Autodesk Inventor part; units mm, degrees
ref_plane "YZ Plane" through (0, 0, 0) normal (1, 0, 0) x (0, 1, 0)
ref_plane "XZ Plane" through (0, 0, 0) normal (0, 1, 0) x (-1, 0, 0)
ref_plane "XY Plane" through (0, 0, 0) normal (0, 0, 1) x (1, 0, 0)
sketch "Эскиз1" plane through (0, 0, 0) normal (0, 1, 0) x (-1, 0, 0)
  line L0 (2.54, -1.27) -> (-2.54, -1.27)
  line L1 (-2.54, -1.27) -> (-2.54, 1.27)
  line L2 (-2.54, 1.27) -> (2.54, 1.27)
  line L3 (2.54, 1.27) -> (2.54, -1.27)
  line L4 (0, -1.778) -> (0, 1.778)
  line L5 (3.556, 0) -> (-3.556, 0)
  point P0 (0, 0)
  dimension "d0" = 5.08
  dimension "d1" = 2.54
extrude "Выдавливание1" add sketch "Эскиз1" along normal blind 6
sketch "Эскиз2" plane through (0, 6, 0) normal (0, 1, 0) x (1, 0, 0)
  line L0 (-1.67, 0.4) -> (-0.87, 0.4)
  line L1 (-0.87, 0.4) -> (-0.87, -0.4)
  line L2 (-0.87, -0.4) -> (-1.67, -0.4)
  line L3 (-1.67, -0.4) -> (-1.67, 0.4)
  line L4 (-3.556, 0) -> (3.556, 0)
  line L5 (0, 1.778) -> (0, -1.778)
  line L6 (0.87, 0.4) -> (1.67, 0.4)
  line L7 (1.67, 0.4) -> (1.67, -0.4)
  line L8 (1.67, -0.4) -> (0.87, -0.4)
  line L9 (0.87, -0.4) -> (0.87, 0.4)
  point P0 (0, 0)
  dimension "d11" = 10
  dimension "d4" = 0.8
  dimension "d5" = 0.8
  dimension "d8" = 2.54
extrude "Выдавливание2" cut sketch "Эскиз2" against normal blind 6
properties part number "jumper"
Source: CAD feature listing. Evaluate the final solid. Frame: model axes, mm. Give positions to 0.01 mm unless a question says otherwise; leave off trailing zeros. Write each loop counter-clockwise with the first axis right and the second up, starting at its lowest first coordinate (ties: lowest second). Pieces come first, ordered by that corner, then holes. Notation, with made-up numbers: M 13,-11.75 L 71,-11.75 A18 cw 71,12.25 Z; hole C 80,-37.75 d11. An arc over 180 degrees is marked long. Answer as a JSON object with one key per item and string values.
Q1. Ray query, line 1 along X through (y, z) = (1.4, 0.05); line 2 along Z through (x, y) = (-1.15, 5.6). Return the intervals inside material, ascending.
Geometry check:
{"line 1": "x = -2.54 to -1.67, -0.87 to 0.87, 1.67 to 2.54", "line 2": "z = -1.27 to -0.4, 0.4 to 1.27"}
Q2. Cut plane B-B, the plane z = -0.05. Return the cut outline in (x, y), then the cut area to 3 significant figures.
Geometry check:
{"outline": "M -2.54,0 L -1.67,0 L -1.67,6 L -2.54,6 Z; M -0.87,0 L 0.87,0 L 0.87,6 L -0.87,6 Z; M 1.67,0 L 2.54,0 L 2.54,6 L 1.67,6 Z", "area": "20.9 mm^2"}
Q3. Cut plane C-C, the plane y = 0.8. Return the cut outline in (x, z), then the cut area to 3 significant figures.
Geometry check:
{"outline": "M -2.54,-1.27 L 2.54,-1.27 L 2.54,1.27 L -2.54,1.27 Z; hole M -1.67,-0.4 L -0.87,-0.4 L -0.87,0.4 L -1.67,0.4 Z; hole M 0.87,-0.4 L 1.67,-0.4 L 1.67,0.4 L 0.87,0.4 Z", "area": "11.6 mm^2"}
Q4. Cut plane A-A, the plane x = 1.55. Return the cut outline in (y, z).
Geometry check:
{"outline": "M 0,-1.27 L 6,-1.27 L 6,-0.4 L 0,-0.4 Z; M 0,0.4 L 6,0.4 L 6,1.27 L 0,1.27 Z"}
